CAD build for the part. Positions are in the model's coordinates, mm. Face numbers are marked on the shaded views. A direction names the side the tool comes from. Give positions to 0.01 mm unless a question says otherwise; leave off trailing zeros. Write each loop counter-clockwise with the first axis right and the second up, starting at its lowest first coordinate (ties: lowest second). Pieces come first, ordered by that corner, then holes. Notation, with made-up numbers: (82, 89) - (139, 89) arc R8 ccw to (139, 97) - close; hole circle Ø6 at (-10.5, 41.5). An arc over 180 degrees is marked (long way). Answer as a JSON object with one key per item and string values.
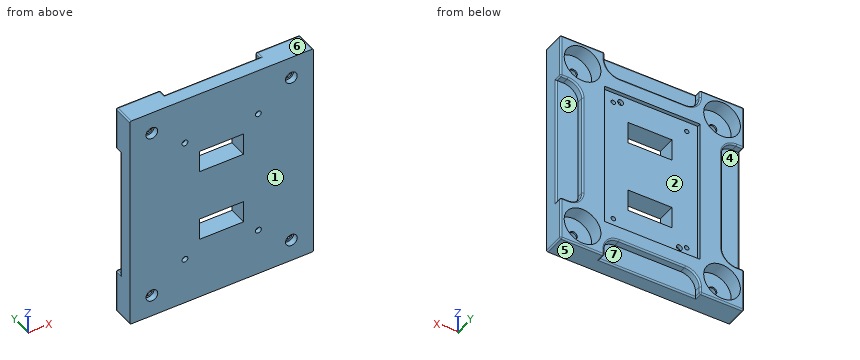
from build123d import *

# Parameters (mm, degrees)
SKETCH1_W                                           = 250
SKETCH1_H                                           = 300
BOSS_EXTRUDE1_DEPTH                                 = 30
SKETCH2_W                                           = 60
SKETCH2_H                                           = 30
CUT_EXTRUDE1_DEPTH                                  = 246
SKETCH4_W                                           = 130
SKETCH4_H                                           = 200
CUT_EXTRUDE2_DEPTH                                  = 5
CBORE_FOR_M5_HEX_SOCKET_HEAD_CAP_SCREW1_D           = 6
CBORE_FOR_M5_HEX_SOCKET_HEAD_CAP_SCREW1_DEPTH       = 30
CBORE_FOR_M5_HEX_SOCKET_HEAD_CAP_SCREW1_CBORE_D     = 8
CBORE_FOR_M5_HEX_SOCKET_HEAD_CAP_SCREW1_CBORE_DEPTH = 6
CBORE_FOR_M5_HEX_SOCKET_HEAD_CAP_SCREW1_TIP         = 1.802581857
CUT_EXTRUDE4_DEPTH                                  = 10
FILLET1_R                                           = 2
FILLET2_R                                           = 2
FILLET3_R                                           = 2
FILLET4_R                                           = 2
FILLET5_R                                           = 2
FILLET7_R                                           = 2
FILLET8_R                                           = 2
FILLET9_R                                           = 2
FILLET10_R                                          = 2
FILLET11_R                                          = 2
FILLET12_R                                          = 2
FILLET13_R                                          = 2
FILLET14_R                                          = 2
FILLET15_R                                          = 2
FILLET16_R                                          = 2
FILLET17_R                                          = 2
SKETCH11_R                                          = 25
CUT_EXTRUDE5_DEPTH                                  = 20
CBORE_FOR_M5_HEX_HEAD_BOLT3_D                       = 11
CBORE_FOR_M5_HEX_HEAD_BOLT3_CBORE_D                 = 16
CBORE_FOR_M5_HEX_HEAD_BOLT3_CBORE_DEPTH             = 8
SKETCH26_R                                          = 4
CUT_EXTRUDE6_DEPTH                                  = 5


with BuildPart() as part:
    # Sketch1 → Boss-Extrude1 (new body)
    with BuildSketch(Plane(origin=(0, 0, 0), x_dir=(1, 0, 0), z_dir=(0, 1, 0))):
        Rectangle(SKETCH1_W, SKETCH1_H)
    extrude(amount=BOSS_EXTRUDE1_DEPTH)

    # Sketch2 → Cut-Extrude1 (cut)
    with BuildSketch(Plane(origin=(0, 30, 0), x_dir=(1, 0, 0), z_dir=(0, 1, 0))):
        with Locations((0, 50)):
            Rectangle(SKETCH2_W, SKETCH2_H)
        with Locations((0, -50)):
            Rectangle(SKETCH2_W, SKETCH2_H)
    extrude(amount=-CUT_EXTRUDE1_DEPTH, mode=Mode.SUBTRACT)

    # Sketch4 → Cut-Extrude2 (cut)
    with BuildSketch(Plane(origin=(0, 30, 0), x_dir=(1, 0, 0), z_dir=(0, 1, 0))):
        Rectangle(SKETCH4_W, SKETCH4_H)
    extrude(amount=-CUT_EXTRUDE2_DEPTH, mode=Mode.SUBTRACT)

    # CBORE for M5 Hex Socket Head Cap Screw1
    with Locations(Plane(origin=(50, 0, -86), x_dir=(0, 0, -1), z_dir=(0, -1, 0))):
        with Locations((0, 0), (0, -100), (-172, -100), (-172, 0)):
            CounterBoreHole(CBORE_FOR_M5_HEX_SOCKET_HEAD_CAP_SCREW1_D / 2, CBORE_FOR_M5_HEX_SOCKET_HEAD_CAP_SCREW1_CBORE_D / 2, CBORE_FOR_M5_HEX_SOCKET_HEAD_CAP_SCREW1_CBORE_DEPTH, depth=CBORE_FOR_M5_HEX_SOCKET_HEAD_CAP_SCREW1_DEPTH)
            with Locations((0, 0, -(CBORE_FOR_M5_HEX_SOCKET_HEAD_CAP_SCREW1_DEPTH + CBORE_FOR_M5_HEX_SOCKET_HEAD_CAP_SCREW1_TIP / 2))):  # 118° drill point
                Cone(0, CBORE_FOR_M5_HEX_SOCKET_HEAD_CAP_SCREW1_D / 2, CBORE_FOR_M5_HEX_SOCKET_HEAD_CAP_SCREW1_TIP, mode=Mode.SUBTRACT)

    # Sketch10 → Cut-Extrude4 (cut)
    with BuildSketch(Plane(origin=(0, 30, 0), x_dir=(1, 0, 0), z_dir=(0, 1, 0))):
        with BuildLine():
            Line((-125, 90), (-115, 90))
            ThreePointArc((-115, 90), (-100.857864376, 84.142135624), (-95, 70))
            Line((-95, 70), (-95, -70))
            ThreePointArc((-95, -70), (-100.857864376, -84.142135624), (-115, -90))
            Line((-115, -90), (-125, -90))
            Line((-125, -90), (-125, 90))
        make_face()
        with BuildLine():
            Line((-65, -150), (65, -150))
            Line((65, -150), (65, -140))
            ThreePointArc((65, -140), (59.142135624, -125.857864376), (45, -120))
            Line((45, -120), (-45, -120))
            ThreePointArc((-45, -120), (-59.142135624, -125.857864376), (-65, -140))
            Line((-65, -140), (-65, -150))
        make_face()
        with BuildLine():
            Line((125, -90), (115, -90))
            ThreePointArc((115, -90), (100.857864376, -84.142135624), (95, -70))
            Line((95, -70), (95, 70))
            ThreePointArc((95, 70), (100.857864376, 84.142135624), (115, 90))
            Line((115, 90), (125, 90))
            Line((125, 90), (125, -90))
        make_face()
        with BuildLine():
            Line((65, 150), (-65, 150))
            Line((-65, 150), (-65, 140))
            ThreePointArc((-65, 140), (-59.142135624, 125.857864376), (-45, 120))
            Line((-45, 120), (45, 120))
            ThreePointArc((45, 120), (59.142135624, 125.857864376), (65, 140))
            Line((65, 140), (65, 150))
        make_face()
    extrude(amount=-CUT_EXTRUDE4_DEPTH, mode=Mode.SUBTRACT)

    # Fillet1
    fillet1_edges = [part.edges().sort_by_distance(p)[0] for p in [
        (-65, 30, 145),
        (65, 30, 145),
        (59.142135624, 30, 125.857864376),
        (0, 30, 120),
        (-59.142135624, 30, 125.857864376),
    ]]
    fillet(fillet1_edges, radius=FILLET1_R)

    # Fillet2
    fillet2_edges = [part.edges().sort_by_distance(p)[0] for p in [
        (-65, 24, 150),
        (-96, 30, 150),
        (-65.585786438, 29.414213562, 150),
    ]]
    fillet(fillet2_edges, radius=FILLET2_R)

    # Fillet3
    fillet3_edges = [part.edges().sort_by_distance(p)[0] for p in [
        (65, 24, 150),
        (96, 30, 150),
        (65.585786438, 29.414213562, 150),
    ]]
    fillet(fillet3_edges, radius=FILLET3_R)

    # Fillet4
    fillet4_edges = [part.edges().sort_by_distance(p)[0] for p in [
        (125, 14, 150),
        (125, 30, 119),
        (125, 29.414213562, 149.414213562),
    ]]
    fillet(fillet4_edges, radius=FILLET4_R)

    # Fillet5
    fillet5_edges = [part.edges().sort_by_distance(p)[0] for p in [
        (125, 24, 90),
        (120, 30, -90),
        (100.857864376, 30, -84.142135624),
        (95, 30, 0),
        (100.857864376, 30, 84.142135624),
        (119, 30, 90),
        (124.414213562, 29.414213562, 90),
    ]]
    fillet(fillet5_edges, radius=FILLET5_R)

    # Fillet7
    fillet7_edges = [part.edges().sort_by_distance(p)[0] for p in [
        (125, 24, -90),
        (125, 30, -121),
        (125, 29.414213562, -90.585786438),
    ]]
    fillet(fillet7_edges, radius=FILLET7_R)

    # Fillet8
    fillet8_edges = [part.edges().sort_by_distance(p)[0] for p in [
        (65, 30, -145),
        (-65, 30, -145),
        (-59.142135624, 30, -125.857864376),
        (0, 30, -120),
        (59.142135624, 30, -125.857864376),
    ]]
    fillet(fillet8_edges, radius=FILLET8_R)

    # Fillet9
    fillet9_edges = [part.edges().sort_by_distance(p)[0] for p in [
        (65, 24, -150),
        (125, 14, -150),
        (95, 30, -150),
        (124.414213562, 29.414213562, -150),
        (65.585786438, 29.414213562, -150),
    ]]
    fillet(fillet9_edges, radius=FILLET9_R)

    # Fillet10
    fillet10_edges = [part.edges().sort_by_distance(p)[0] for p in [
        (-65, 24, -150),
        (-96, 30, -150),
        (-65.585786438, 29.414213562, -150),
    ]]
    fillet(fillet10_edges, radius=FILLET10_R)

    # Fillet11
    fillet11_edges = [part.edges().sort_by_distance(p)[0] for p in [
        (-125, 14, -150),
        (-125, 30, -119),
        (-125, 29.414213562, -149.414213562),
    ]]
    fillet(fillet11_edges, radius=FILLET11_R)

    # Fillet12
    fillet12_edges = [part.edges().sort_by_distance(p)[0] for p in [
        (-125, 24, -90),
        (-120, 30, 90),
        (-100.857864376, 30, 84.142135624),
        (-95, 30, 0),
        (-100.857864376, 30, -84.142135624),
        (-119, 30, -90),
        (-124.414213562, 29.414213562, -90),
    ]]
    fillet(fillet12_edges, radius=FILLET12_R)

    # Fillet13
    fillet13_edges = [part.edges().sort_by_distance(p)[0] for p in [
        (-125, 24, 90),
        (-125, 14, 150),
        (-125, 29.414213562, 149.414213562),
        (-125, 30, 120),
        (-125, 29.414213562, 90.585786438),
    ]]
    fillet(fillet13_edges, radius=FILLET13_R)

    # Fillet14
    fillet14_edges = [part.edges().sort_by_distance(p)[0] for p in [
        (-125, 20, 0),
    ]]
    fillet(fillet14_edges, radius=FILLET14_R)

    # Fillet15
    fillet15_edges = [part.edges().sort_by_distance(p)[0] for p in [
        (0, 20, 150),
    ]]
    fillet(fillet15_edges, radius=FILLET15_R)

    # Fillet16
    fillet16_edges = [part.edges().sort_by_distance(p)[0] for p in [
        (125, 20, 0),
    ]]
    fillet(fillet16_edges, radius=FILLET16_R)

    # Fillet17
    fillet17_edges = [part.edges().sort_by_distance(p)[0] for p in [
        (0, 20, -150),
    ]]
    fillet(fillet17_edges, radius=FILLET17_R)

    # Sketch11 → Cut-Extrude5 (cut)
    with BuildSketch(Plane(origin=(0, 30, 0), x_dir=(1, 0, 0), z_dir=(0, 1, 0))):
        with Locations((-95, 120)):
            Circle(SKETCH11_R)
        with Locations((95, 120)):
            Circle(SKETCH11_R)
        with Locations((95, -120)):
            Circle(SKETCH11_R)
        with Locations((-95, -120)):
            Circle(SKETCH11_R)
    extrude(amount=-CUT_EXTRUDE5_DEPTH, mode=Mode.SUBTRACT)

    # CBORE for M5 Hex Head Bolt3 (through all)
    with Locations(Plane(origin=(95, 0, -120), x_dir=(0, 0, -1), z_dir=(0, -1, 0))):
        with Locations((0, 0), (0, -190), (-240, -190), (-240, 0)):
            CounterBoreHole(CBORE_FOR_M5_HEX_HEAD_BOLT3_D / 2, CBORE_FOR_M5_HEX_HEAD_BOLT3_CBORE_D / 2, CBORE_FOR_M5_HEX_HEAD_BOLT3_CBORE_DEPTH)

    # Sketch26 → Cut-Extrude6 (cut)
    with BuildSketch(Plane(origin=(0, 25, 0), x_dir=(1, 0, 0), z_dir=(0, 1, 0))):
        with Locations((40, -90)):
            Circle(SKETCH26_R)
        with Locations((-40, 90)):
            Circle(SKETCH26_R)
    extrude(amount=-CUT_EXTRUDE6_DEPTH, mode=Mode.SUBTRACT)


solid = part.part
Item 1: Flat gauge pins, fed straight in: P1, Ø12, axis at y = 18.5, z = 70.5, coming from the -X side; P2, Ø1.5, axis at x = 31.5, y = 26, coming from the -Z side; P3, Ø6, axis at y = 25, z = -65, coming from the +X side; P4, Ø5.5, axis at y = 27, z = 10.5, coming from the -X side. Where does each tip first touch, or does it go through?
Entries:
{"P1": "x = -125", "P2": "z = -120", "P3": "x = 95", "P4": "x = -95"}
Item 2: Probe line 1 (Z direction, x = 10, y = 14); line 2 (Z direction, x = 110, y = 11.5); line 3 (X direction, y = 15, z = -120). List the from-to ranges inside material, lowest first. Write a range as from..to.
Entries:
{"line 1": "-150..-65, -35..35, 65..150", "line 2": "-150..-140, -100..100, 140..150", "line 3": "-125..-120, -70..70, 120..125"}
Item 3: Which spindle directions (+Z, -Z, +X, -X, +Y, -Y) get a long thin tool onto all of the face, cutting with end or side? Do the marked faces 3, 4, 5, 6 and 7. Say none if no direction does.
Entries:
{"face 3": "+X, +Y", "face 4": "-X, +Y", "face 5": "-Z, +X, -X, +Y, -Y", "face 6": "+Z, +X, -X, +Y, -Y", "face 7": "-Z, +Y"}
Item 4: Mould opens along X. For the marked faces 1 and 2 say: +X half, -X half, draft (parallel to the pull), parting line (faces both ways), or undercut.
Entries:
{"face 1": "draft", "face 2": "undercut"}
Item 5: Cut at A-A (x = 9). Give the cut face in (y, z), and give its area (3 significant figures).
Entries:
{"outline": "(0, -150) - (18, -150) arc R2 ccw to (20, -148) - (20, -120) - (28, -120) arc R2 ccw to (30, -118) - (30, -100) - (25, -100) - (25, -65) - (0, -65) - close; (0, -35) - (25, -35) - (25, 35) - (0, 35) - close; (0, 65) - (25, 65) - (25, 100) - (30, 100) - (30, 118) arc R2 ccw to (28, 120) - (20, 120) - (20, 148) arc R2 ccw to (18, 150) - (0, 150) - close", "area": "5,900 mm2"}
Item 6: Cut at C-C (x = 40). Give the cut face in (y, z).
Entries:
{"outline": "(0, -150) - (18, -150) arc R2 ccw to (20, -148) - (20, -120) - (28, -120) arc R2 ccw to (30, -118) - (30, -100) - (25, -100) - (25, 86) - (20, 86) - (20, 94) - (25, 94) - (25, 100) - (30, 100) - (30, 118) arc R2 ccw to (28, 120) - (20, 120) - (20, 148) arc R2 ccw to (18, 150) - (0, 150) - close"}
Item 7: Cut at B-B (z = 22.5). Give the cut face in (x, y), and give its area (3 significant figures).
Entries:
{"outline": "(-125, 0) - (125, 0) - (125, 18) arc R2 ccw to (123, 20) - (95, 20) - (95, 28) arc R2 ccw to (93, 30) - (65, 30) - (65, 25) - (-65, 25) - (-65, 30) - (-93, 30) arc R2 ccw to (-95, 28) - (-95, 20) - (-123, 20) arc R2 ccw to (-125, 18) - close", "area": "6,250 mm2"}
